```python
from build123d import *

# Parameters (mm, degrees)
F0_R      = 0.635
F1_DEPTH  = 3.81
F2_R      = 0.635
F3_DEPTH  = 0.254
F5_DEPTH  = 1.524
F7_DEPTH  = 1.524
F9_R      = 1.016
F10_DEPTH = 6.604
F0_R_2    = 1.27
F11_DEPTH = 1.27
F12_R     = 1.27


# Not quite as in the source:
# - two fillets or chamfers of one size are made in one step
# - a pattern or mirror of a feature is missing from the dataset's text; its kind, count and spacing are read off the source's solid


with BuildPart() as f1:
    # F0 (on Front) → F1 (new body)
    with BuildSketch(Plane.XZ):
        with BuildLine():
            Line((6.35, 50.8), (0, 57.15))
            Line((0, 57.15), (0, 0))
            Line((0, 0), (2.032, 0))
            Line((2.032, 0), (4.4819667348, 5.2539706179))
            Line((4.4819667348, 5.2539706179), (5.8556178921, 15.0280064712))
            ThreePointArc((5.8556178921, 15.0280064712), (6.2262537532, 18.5543711338), (6.35, 22.098))
            Line((6.35, 22.098), (6.35, 50.8))
        make_face()
        with Locations((2.032, 12.7)):
            Circle(F0_R, mode=Mode.SUBTRACT)
    extrude(amount=-F1_DEPTH)

    # F1_copies: F1 across plane


with BuildPart() as f1_1:
    add(f1.part)
    add(f1.part.mirror(Plane(origin=(0, 0, 0), x_dir=(0, 0, -1), z_dir=(0, -1, 0))))

    # F2 (on face) → F3 (cut)
    with BuildSketch(Plane.XZ):
        with BuildLine():
            Line((6.35, 31.75), (0, 31.75))
            Line((0, 31.75), (0, 0))
            Line((0, 0), (2.032, 0))
            Line((2.032, 0), (4.4819667348, 5.2539706179))
            Line((4.4819667348, 5.2539706179), (5.8556178921, 15.0280064712))
            ThreePointArc((5.8556178921, 15.0280064712), (6.2262537532, 18.5543711338), (6.35, 22.098))
            Line((6.35, 22.098), (6.35, 31.75))
        make_face()
        with Locations((2.032, 12.7)):
            Circle(F2_R, mode=Mode.SUBTRACT)
    f3 = extrude(amount=-F3_DEPTH, mode=Mode.SUBTRACT)

    # F3_copies: F3 across plane
    add(f3.mirror(Plane(origin=(0, 0, 0), x_dir=(0, 0, -1), z_dir=(0, -1, 0))), mode=Mode.SUBTRACT)

    # F4 (on Front) → F5 (cut, symmetric)
    with BuildSketch(Plane.XZ):
        with BuildLine():
            Line((4.4819667348, 5.2539706179), (4.8144904791, 7.62))
            Line((4.8144904791, 7.62), (5.8556178921, 15.0280064712))
            ThreePointArc((5.8556178921, 15.0280064712), (6.0717122847, 16.787954066), (6.2262537532, 18.5543711338))
            ThreePointArc((6.2262537532, 18.5543711338), (2.8470783684, 12.2329567007), (4.4819667348, 5.2539706179))
        make_face()
        with BuildLine():
            Line((5.8556178921, 15.0280064712), (4.8144904791, 7.62))
            Line((4.8144904791, 7.62), (4.4819667348, 5.2539706179))
            Line((4.4819667348, 5.2539706179), (6.2262537532, 5.0006376953))
            Line((6.2262537532, 5.0006376953), (8.3210639079, 18.5543711338))
            Line((8.3210639079, 18.5543711338), (6.2262537532, 18.5543711338))
            ThreePointArc((6.2262537532, 18.5543711338), (6.0717122847, 16.787954066), (5.8556178921, 15.0280064712))
        make_face()
    extrude(amount=F5_DEPTH, both=True, mode=Mode.SUBTRACT)

    # F4 (on Front) → F7 (cut, symmetric)
    with BuildSketch(Plane.XZ):
        with BuildLine():
            Line((4.4819667348, 5.2539706179), (4.8144904791, 7.62))
            Line((4.8144904791, 7.62), (5.8556178921, 15.0280064712))
            ThreePointArc((5.8556178921, 15.0280064712), (6.0717122847, 16.787954066), (6.2262537532, 18.5543711338))
            ThreePointArc((6.2262537532, 18.5543711338), (2.8470783684, 12.2329567007), (4.4819667348, 5.2539706179))
        make_face()
        with BuildLine():
            Line((5.8556178921, 15.0280064712), (4.8144904791, 7.62))
            Line((4.8144904791, 7.62), (4.4819667348, 5.2539706179))
            Line((4.4819667348, 5.2539706179), (6.2262537532, 5.0006376953))
            Line((6.2262537532, 5.0006376953), (8.3210639079, 18.5543711338))
            Line((8.3210639079, 18.5543711338), (6.2262537532, 18.5543711338))
            ThreePointArc((6.2262537532, 18.5543711338), (6.0717122847, 16.787954066), (5.8556178921, 15.0280064712))
        make_face()
    extrude(amount=F7_DEPTH, both=True, mode=Mode.SUBTRACT)

    # F9 (on face) → F10 (cut)
    with BuildSketch(Plane(origin=(0, 0, 0), x_dir=(0.9747835757, 0, -0.2231523707), z_dir=(0.2231523707, 0, 0.9747835757))):
        with Locations((1.016, 0)):
            Circle(F9_R)
    extrude(amount=F10_DEPTH, mode=Mode.SUBTRACT)

    # F0 (on Front) → F11 (join, symmetric)
    with BuildSketch(Plane.XZ):
        Polygon((0, 66.802), (0, 57.15), (6.35, 50.8), (6.35, 60.452), align=None)
        with Locations((2.54, 61.468)):
            Circle(F0_R_2, mode=Mode.SUBTRACT)
    extrude(amount=F11_DEPTH, both=True)

    # F12 (call 1 of 2: OpenCascade refuses the feature's edges together)
    f12_edges = [f1_1.edges().sort_by_distance(p)[0] for p in [
        (1.016, 3.81, 0),
        (6.35, 3.81, 36.449),
        (6.226254, 3.81, 18.554371),
        (3.256983, 3.81, 2.626985),
        (5.168792, 3.81, 10.140989),
        (2.032, 2.06429, 0),
    ]]
    fillet(f12_edges, radius=F12_R)

    # F12#2 (call 2 of 2)
    f12_2_edges = [f1_1.edges().sort_by_distance(p)[0] for p in [
        (6.35, -3.81, 36.449),
        (1.016, -3.81, 0),
        (3.256983, -3.81, 2.626985),
        (5.168792, -3.81, 10.140989),
        (6.226254, -3.81, 18.554371),
        (2.032, -2.06429, 0),
    ]]
    fillet(f12_2_edges, radius=F12_R)


solid = f1_1.part
```
Design review of the part built by this model. Coordinates are the model's own, in mm. A direction names the side the tool comes from. Round coordinates to 2 decimals unless told otherwise and drop trailing zeros. Order: outer loops, then holes, each group sorted by start corner. A loop starts at its lowest first (then second) coordinate and runs counter-clockwise, first axis right, second up. Notation, with made-up numbers: (55.5, 26.5) - (74.5, 26.5) arc R23 cw to (74.5, 41.5) - close; hole circle Ø2 at (4, -36). An arc over 180 degrees is marked (long way). Return JSON: item names as keys, results as strings.
Q1. Consider section B-B on z = 54. Write out the cut boundary in (x, y), plus the area to 3 significant figures.
Computed values:
{"outline": "(0, -3.81) - (3.15, -3.81) - (3.15, -1.27) - (6.35, -1.27) - (6.35, 1.27) - (3.15, 1.27) - (3.15, 3.81) - (0, 3.81) - close", "area": "32.1 mm2"}
Q2. For pin 1 Ø1.9 at (x, z) = (4, 60.5) entering from +Y; pin 2 Ø3.5 at (x, z) = (2.54, 61.468) entering from -Y; pin 3 Ø1 at (y, z) = (0.5, 18) entering from +X, all flat-tipped, find the tip position at first contact; note any pin that passes through.
Computed values:
{"pin 1": "stops at y = 1.27", "pin 2": "stops at y = -1.27", "pin 3": "stops at x = 6.16"}
Q3. Machinability: for faces 1 (the flat face through (2, 0.254, 20)), 2 (the cylindrical face through (2.86, -0.9, 12.33)), 3 (the flat face through (3, 1.27, 59)), which of the approach directions +Z, -Z, +X, -X, +Y, -Y give a long, thin tool a straight path to every point of the face, cutting with its end or side? Answer none if there is none.
Computed values:
{"face 1": "-Z, +X, -X", "face 2": "+X", "face 3": "+Z, +X, +Y"}
Q4. Consider section C-C on z = 12.7. Give the number of separate pieces and of enclosed holes in the cut face, plus the area to 3 significant figures.
Computed values:
{"separate pieces": "4", "enclosed holes": "0", "area": "23.0 mm2"}
Q5. Wall thickness on L1, parallel to Y at x = 2, z = 20; L2, parallel to X at y = 1.25, z = 21.5; L3, parallel to Z at x = 2.54, y = 0: over which ranges is each line inside the solid? List them lowest first. Write a range as [from, to].
Computed values:
{"L1": "y = [-3.81, -0.25], [0.25, 3.81]", "L2": "x = [0, 6.35]", "L3": "z = [31.75, 60.2], [62.74, 64.26]"}
Q6. The part is to be moulded in two halves that separate along Y. For faces 4 (the cylindrical face through (5.988, 3.428, 37.294)), 5 (the flat face through (2, -0.254, 20)), 6 (the flat face through (5.16, -2.02, 10.07)), say which applies: pulls with the +Y half, pulls with the -Y half, needs draft (parallel to the pull), parting line crosses it, or undercut.
Computed values:
{"face 4": "pulls with the +Y half", "face 5": "undercut", "face 6": "needs draft"}
Q7. Consider section A-A on z = 28.5. Write out the cut boundary in (x, y), plus the area to 3 significant figures.
Computed values:
{"outline": "(0, -3.81) - (5.08, -3.81) arc R1.27 ccw to (6.35, -2.54) - (6.35, -0.25) - (0, -0.25) - close; (0, 0.25) - (6.35, 0.25) - (6.35, 2.54) arc R1.27 ccw to (5.08, 3.81) - (0, 3.81) - close", "area": "44.5 mm2"}
